from build123d import *

# Parameters (mm, degrees)
F0_R             = 8
F1_DEPTH         = 6
F3_DEPTH         = 2
F4_R             = 2
F5_DEPTH         = 1
F7_R             = 5.5
F8_DEPTH         = 22
F9_R             = 6.5
F9_R_2           = 5.5
F10_DEPTH        = 10
F11_SIZE         = 1
F12_W            = 1
F12_H            = 2
F13_DEPTH        = 20
F13_COPIES_COUNT = 18


# Not quite as in the source:
# - a fillet or chamfer that OpenCascade refuses, or shapes differently, is made with other operations: its cross-section is extruded or revolved along the edge and cut away or added
# - a pattern or mirror of a feature is missing from the dataset's text; its kind, count and spacing are read off the source's solid


with BuildPart() as f1:
    # F0 (on Front) → F1 (new body)
    with BuildSketch(Plane.XZ):
        Circle(F0_R)
    extrude(amount=-F1_DEPTH)

    # F2 (on face) → F3 (join)
    with BuildSketch(Plane.XZ):
        Polygon((-1.7320508076, 3), (-3.4641016151, 0), (-1.7320508076, -3), (1.7320508076, -3), (3.4641016151, 0), (1.7320508076, 3), align=None)
    extrude(amount=F3_DEPTH)

    # F4 (on face) → F5 (join)
    with BuildSketch(Plane.XZ.offset(2)):
        Circle(F4_R)
    extrude(amount=F5_DEPTH)

    # F6: fillet of radius 2 on 1 edges, made by hand

    # F6_s1 → F6_t2 (revolve, cut)
    with BuildSketch(Plane.XY):
        with BuildLine():
            ThreePointArc((2, -2), (1.2679491924, -2.7320508076), (0.2679491924, -3))
            Line((0.2679491924, -3), (2, -3))
            Line((2, -3), (2, -2))
        make_face()
    revolve(axis=Axis((0, -3, 0), (0, -1, 0)), mode=Mode.SUBTRACT)

    # F7 (on face) → F8 (join)
    with BuildSketch(Plane(origin=(0, 6, 0), x_dir=(-1, 0, 0), z_dir=(0, 1, 0))):
        Circle(F7_R)
    extrude(amount=F8_DEPTH)

    # F9 (on face) → F10 (join)
    with BuildSketch(Plane(origin=(0, 28, 0), x_dir=(-1, 0, 0), z_dir=(0, 1, 0))):
        Circle(F9_R)
        Circle(F9_R_2, mode=Mode.SUBTRACT)
    extrude(amount=-F10_DEPTH)

    # F11
    f11_edges = [f1.edges().sort_by_distance(p)[0] for p in [
        (6.5, 28, 0),
    ]]
    chamfer(f11_edges, length=F11_SIZE)

    # F12 (on face) → F13 (cut)
    with BuildSketch(Plane(origin=(0, 28, 0), x_dir=(-1, 0, 0), z_dir=(0, 1, 0))):
        with Locations((0, 6.7)):
            Rectangle(F12_W, F12_H)
    f13 = extrude(amount=-F13_DEPTH, mode=Mode.SUBTRACT)

    # F13_copies: F13 ×18 about axis
    f13_copies_axis = Axis((0, 0, 0), (0, 1, 0))
    for i in range(1, F13_COPIES_COUNT):
        add(f13.rotate(f13_copies_axis, i * 360 / F13_COPIES_COUNT), mode=Mode.SUBTRACT)


solid = f1.part
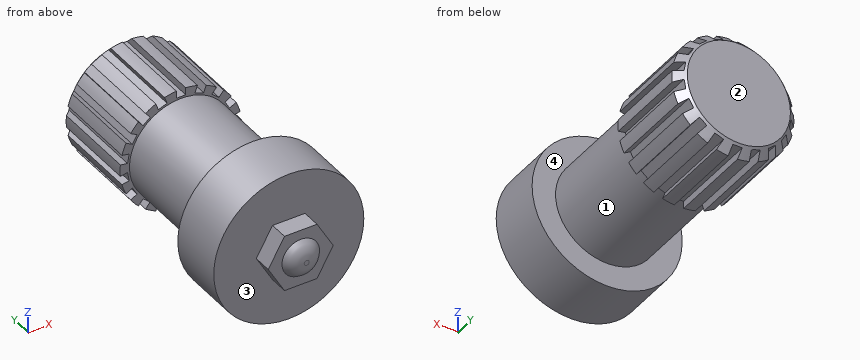
Geometry: final body of the model. Coordinates: model frame, mm. Face numbers are marked on the shaded views. Give positions to 0.01 mm unless a question says otherwise; leave off trailing zeros. Write each loop counter-clockwise with the first axis right and the second up, starting at its lowest first coordinate (ties: lowest second). Pieces come first, ordered by that corner, then holes.
(1) First-contact query: P1, Ø6, axis at y = 17, z = 4.5, coming from the +X side; P2, Ø0.6, axis at x = -0.5, y = -1, coming from the -Z side; P3, Ø0.9, axis at y = 25.5, z = 6, coming from the -X side. Flat tips, straight axial feed; report the tip coordinate or a pass-through.
(2) Cut plane A-A, the plane y = 15. Return loops of the section in (x, z), then the cut area to 3 significant figures.
(3) Mould query, pull axis Y, two halves, no side actions, for the marked faces 1, 2, 3 and 4. Classes: released by +Y, released by -Y, zero draft, split by the parting line, or undercut.
(4) Ray query, line 1 (X direction, y = 20, z = 4.5); line 2 (Y direction, x = 3, z = -7); line 3 (X direction, y = 22, z = 1.75). Return the intervals inside material, ascending.
Values follow:
1. P1: stops at x = 6.28
1. P2: stops at z = -3
1. P3: stops at x = -3.38
2. outline: circle Ø11 at (0, 0)
2. area: 95.0 mm2
3. face 1: undercut
3. face 2: released by +Y
3. face 3: released by -Y
3. face 4: undercut
4. line 1: x = -4.69 to -4.43, -3.5 to 3.5, 4.43 to 4.69
4. line 2: y = 0 to 6
4. line 3: x = -6.26 to 6.26
